For this review, take the finished solid that the model builds, in its own axes (mm). Face numbers are marked on the shaded views. A direction names the side the tool comes from. Give positions to 0.01 mm unless a question says otherwise; leave off trailing zeros. Loops run counter-clockwise (first coordinate to the right, second up) from the corner with the lowest first, then second, coordinate; pieces in that order, holes last.
```python
from build123d import *

# Parameters (mm, degrees)
F0_W     = 24.4314651938
F0_H     = 83.410562446
F0_R     = 9.271
F0_W_2   = 103.4520039098
F0_H_2   = 21.7592747342
F1_DEPTH = 76.2
F3_DEPTH = 172.974
F4_DEPTH = 21.59
F6_DEPTH = 21.59


with BuildPart() as f1:
    # F0 (on Top) → F1 (new body)
    with BuildSketch(Plane.XY):
        with Locations((63.9417345518, 0)):
            Rectangle(F0_W, F0_H)
        with Locations((64.3234781713, 0)):
            Circle(F0_R, mode=Mode.SUBTRACT)
        Rectangle(F0_W_2, F0_H)
        with Locations((0, 52.5849185901)):
            Rectangle(F0_W_2, F0_H_2)
        with Locations((-63.9417345518, 0)):
            Rectangle(F0_W, F0_H)
        with Locations((-64.3234781713, 0)):
            Circle(F0_R, mode=Mode.SUBTRACT)
        with Locations((0, -52.5849185901)):
            Rectangle(F0_W_2, F0_H_2)
    extrude(amount=F1_DEPTH)

    # F2 (on face) → F3 (cut)
    with BuildSketch(Plane.XZ.offset(63.4645559572)):
        with BuildLine():
            Line((33.6816743844, 76.2), (-33.6816743844, 76.2))
            ThreePointArc((-33.6816743844, 76.2), (0, 42.5183256156), (33.6816743844, 76.2))
        make_face()
    extrude(amount=-F3_DEPTH, mode=Mode.SUBTRACT)

    # F2 (on face) → F4 (cut)
    with BuildSketch(Plane.XZ.offset(63.4645559572)):
        with BuildLine():
            ThreePointArc((51.6462088302, 76.2), (0, 24.5537911698), (-51.6462088302, 76.2))
            Line((-51.6462088302, 76.2), (-51.7260019549, 76.2))
            Line((-51.7260019549, 76.2), (-51.7260019549, 0))
            Line((-51.7260019549, 0), (51.7260019549, 0))
            Line((51.7260019549, 0), (51.7260019549, 76.2))
            Line((51.7260019549, 76.2), (51.6462088302, 76.2))
        make_face()
    extrude(amount=-F4_DEPTH, mode=Mode.SUBTRACT)

    # F5 (on face) → F6 (cut)
    with BuildSketch(Plane(origin=(0, 63.4645559572, 0), x_dir=(-1, 0, 0), z_dir=(0, 1, 0))):
        with BuildLine():
            ThreePointArc((51.7260019549, 76.2), (0, 24.4739980451), (-51.7260019549, 76.2))
            Line((-51.7260019549, 76.2), (-51.7260019549, 0))
            Line((-51.7260019549, 0), (51.7260019549, 0))
            Line((51.7260019549, 0), (51.7260019549, 76.2))
        make_face()
    extrude(amount=-F6_DEPTH, mode=Mode.SUBTRACT)


solid = f1.part
```
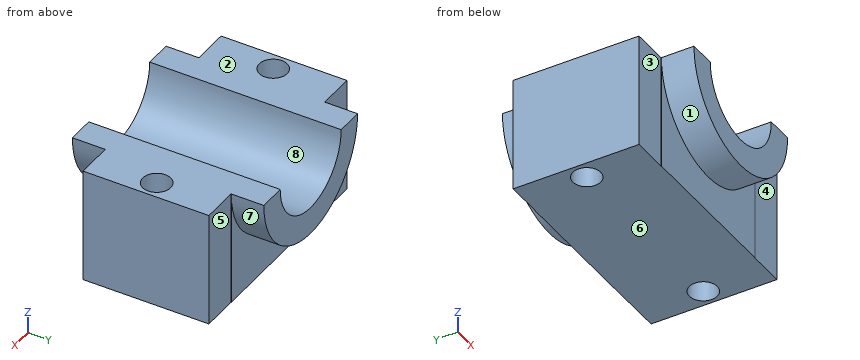
Q1. Consider section B-B on z = 6. Give the boundary of the cut face in (x, y), plus the area to 3 significant figures.
Answers:
outline: (-76.16, -41.71) - (-51.73, -41.71) - (-51.73, -41.87) - (51.73, -41.87) - (51.73, -41.71) - (76.16, -41.71) - (76.16, 41.71) - (51.73, 41.71) - (51.73, 41.87) - (-51.73, 41.87) - (-51.73, 41.71) - (-76.16, 41.71) - close; hole circle Ø18.54 at (-64.32, 0); hole circle Ø18.54 at (64.32, 0)
area: 12,200 mm2
Q2. Machinability: for the marked faces 1, 2, 3, 4 and 5, which of the approach directions +Z, -Z, +X, -X, +Y, -Y give a long, thin tool a straight path to every point of the face, cutting with its end or side? Answer none if there is none.
Answers:
face 1: -Z, -Y
face 2: +Z, +X, -X, +Y, -Y
face 3: +Z, -Z, -X, -Y
face 4: +Z, -Z, +X, -Y
face 5: +Z, -Z, +X, +Y
Q3. Consider section A-A on y = 0. Give the boundary of the cut face in (x, z), plus the area to 3 significant figures.
Answers:
outline: (-76.16, 0) - (-73.59, 0) - (-73.59, 76.2) - (-76.16, 76.2) - close; (-55.05, 0) - (55.05, 0) - (55.05, 76.2) - (33.68, 76.2) arc R33.68 cw to (-33.68, 76.2) - (-55.05, 76.2) - close; (73.59, 0) - (76.16, 0) - (76.16, 76.2) - (73.59, 76.2) - close
area: 7,000 mm2
Q4. Consider section C-C on x = -63. Give the boundary of the cut face in (y, z).
Answers:
outline: (-41.71, 0) - (-9.18, 0) - (-9.18, 76.2) - (-41.71, 76.2) - close; (9.18, 0) - (41.71, 0) - (41.71, 76.2) - (9.18, 76.2) - close
Q5. For pin 1 Ø4 at (x, z) = (-31, 26) entering from -Y; pin 2 Ø2 at (x, y) = (-41.5, -40.5) entering from -Z; pin 3 Ø16.5 at (x, y) = (-64.32, 0) entering from +Z; pin 4 Ø1.5 at (x, y) = (4, 32) entering from +Z, all flat-tipped, find the tip position at first contact; note any pin that passes through.
Answers:
pin 1: stops at y = -41.87
pin 2: stops at z = 0
pin 3: passes through
pin 4: stops at z = 42.85
Q6. Consider section D-D on x = 0. Give the boundary of the cut face in (y, z).
Answers:
outline: (-63.46, 24.55) - (-41.87, 24.55) - (-41.87, 0) - (41.87, 0) - (41.87, 24.47) - (63.46, 24.47) - (63.46, 42.52) - (-63.46, 42.52) - close
Q7. Mouldability with a two-part tool opening along X and no side actions: class the marked faces 6, 7 and 8 as +X half, -X half, draft (parallel to the pull), parting line (faces both ways), or undercut.
Answers:
face 6: draft
face 7: parting line
face 8: undercut
Q8. For probe 1 along Y at (x, z) = (32, 14); probe 2 along Y at (x, z) = (68, 65); probe 3 along X at (y, z) = (-38, 53.5), list the stretches that pass through material, from the lowest coordinate up.
Answers:
probe 1: y = -41.87 to 41.87
probe 2: y = -41.71 to -8.51, 8.51 to 41.71
probe 3: x = -76.16 to -24.88, 24.88 to 76.16
